from build123d import *

# Parameters (mm, degrees)
SKETCH1_W           = 70.104
SKETCH1_H           = 14.986
BOSS_EXTRUDE1_DEPTH = 21.9964
CUT_EXTRUDE1_DEPTH  = 75.986616306
SKETCH4_R           = 1.5
CUT_EXTRUDE2_DEPTH  = 75.986616306
SKETCH5_R           = 1.27
BOSS_EXTRUDE2_DEPTH = 17.272
BOSS_EXTRUDE3_DEPTH = 14.986
SKETCH7_W           = 11.9888
SKETCH7_H           = 21.9964
BOSS_EXTRUDE4_DEPTH = 0.508
BOSS_EXTRUDE4_TAPER = 45


with BuildPart() as part:
    # Sketch1 → Boss-Extrude1 (new body)
    with BuildSketch(Plane(origin=(0, 0, 0), x_dir=(1, 0, 0), z_dir=(0, 1, 0))):
        with Locations((-35.052, 7.493)):
            Rectangle(SKETCH1_W, SKETCH1_H)
    extrude(amount=BOSS_EXTRUDE1_DEPTH)

    # Sketch3 → Cut-Extrude1 (cut, through all)
    with BuildSketch(Plane.XY):
        with BuildLine():
            Line((-29.337, 13.735160497), (-40.767, 13.735160497))
            ThreePointArc((-40.767, 13.735160497), (-58.1152, 10.9982), (-40.767, 8.261239503))
            Line((-40.767, 8.261239503), (-29.337, 8.261239503))
            ThreePointArc((-29.337, 8.261239503), (-11.9888, 10.9982), (-29.337, 13.735160497))
        make_face()
        Polygon((-58.1152, 21.9964), (-55.5752, 21.3614), (-14.5288, 21.3614), (-11.9888, 21.9964), align=None)
        Polygon((-58.1152, 0), (-55.5752, 0.635), (-14.5288, 0.635), (-11.9888, 0), align=None)
    extrude(amount=-CUT_EXTRUDE1_DEPTH, mode=Mode.SUBTRACT)

    # Sketch4 → Cut-Extrude2 (cut, through all)
    with BuildSketch(Plane(origin=(0, 21.9964, 0), x_dir=(1, 0, 0), z_dir=(0, 1, 0))):
        with Locations(Location((-64.0588, 10.9982, 0), (0, 0, 270))):
            Circle(SKETCH4_R)
        with Locations(Location((-64.0588, 3.9878, 0), (0, 0, 270))):
            Circle(SKETCH4_R)
        with Locations(Location((-6.0452, 3.9878, 0), (0, 0, 90))):
            Circle(SKETCH4_R)
        with Locations(Location((-6.0452, 10.9982, 0), (0, 0, 90))):
            Circle(SKETCH4_R)
    extrude(amount=-CUT_EXTRUDE2_DEPTH, mode=Mode.SUBTRACT)

    # Sketch5 → Boss-Extrude2 (add)
    with BuildSketch(Plane(origin=(0, 0, 0), x_dir=(0, 0, -1), z_dir=(1, 0, 0))):
        with Locations(Location((7.493, 3.23214606, 0), (0, 0, 180))):
            Circle(SKETCH5_R)
    extrude(amount=BOSS_EXTRUDE2_DEPTH)

    # Sketch6 → Boss-Extrude3 (add, through all)
    with BuildSketch(Plane.XY):
        Polygon((-58.1152, 21.9964), (-55.5752, 21.3614), (-14.5288, 21.3614), (-11.9888, 21.9964), (-14.5288, 22.6314), (-55.5752, 22.6314), align=None)
        Polygon((-55.5752, -0.635), (-14.5288, -0.635), (-11.9888, 0), (-14.5288, 0.635), (-55.5752, 0.635), (-58.1152, 0), align=None)
    extrude(amount=-BOSS_EXTRUDE3_DEPTH)

    # Sketch7 → Boss-Extrude4 (add)
    with BuildSketch(Plane(origin=(0, 0, -14.986), x_dir=(-1, 0, 0), z_dir=(0, 0, -1))):
        with Locations((5.9944, 10.9982)):
            Rectangle(SKETCH7_W, SKETCH7_H)
    extrude(amount=BOSS_EXTRUDE4_DEPTH, taper=BOSS_EXTRUDE4_TAPER)


solid = part.part
Geometry: final body of the model. Coordinates: model frame, mm. A direction names the side the tool comes from. Coordinates: 2 decimals unless noted, no trailing zeros. Order: outer loops, then holes, each group sorted by start corner. A loop starts at its lowest first (then second) coordinate and runs counter-clockwise, first axis right, second up.
1) Section A-A (z = -11). Return loops of the section in (x, y) (3 decimals), then the cut area to 3 significant figures.
Result sheet:
outline: (-70.104, 0) - (-65.559, 0) - (-65.559, 21.996) - (-70.104, 21.996) - close; (-62.559, 0) - (-58.115, 0) - (-55.575, -0.635) - (-14.529, -0.635) - (-11.989, 0) - (-7.545, 0) - (-7.545, 21.996) - (-11.989, 21.996) - (-14.529, 22.631) - (-55.575, 22.631) - (-58.115, 21.996) - (-62.559, 21.996) - close; (-4.545, 0) - (0, 0) - (0, 21.996) - (-4.545, 21.996) - close; hole (-40.767, 8.261) - (-29.337, 8.261) arc R8.89 ccw (long way) to (-29.337, 13.735) - (-40.767, 13.735) arc R8.89 ccw (long way) to start
area: 909 mm2
2) Ray query, probe 1 along Z at (x, y) = (-6, 17); probe 2 along X at (y, z) = (20.75, -3.25); probe 3 along Z at (x, y) = (-64.5, 11.5). Return the intervals inside material, ascending.
Result sheet:
probe 1: z = -15.49 to -12.5, -9.5 to -5.49, -2.49 to 0
probe 2: x = -70.1 to -65.36, -62.75 to -7.35, -4.74 to 0
probe 3: z = -14.99 to -12.43, -9.56 to -5.42, -2.55 to 0
3) Set-up query: faces 1 (the flat face through (-6, 21.996, -8)), 2 (the flat face through (-6, 0, -8)), 3 (the flat face through (-64, 0, -8)), 4 (the flat face through (-41, 16, -14.986)), 5 (the flat face through (-35, 8.261, -7)). Return all of +Z, -Z, +X, -X, +Y, -Y with unobstructed straight access to the full face (end or side cutting, diameter ignored); none if empty.
Result sheet:
face 1: +Z, -Z, +X, +Y
face 2: +Z, -Z, +X, -Y
face 3: +Z, -Z, -X, -Y
face 4: -Z, -X, +Y, -Y
face 5: +Z, -Z
4) Section B-B (x = -34). Return loops of the section in (y, z) (3 decimals).
Result sheet:
outline: (-0.635, -14.986) - (8.261, -14.986) - (8.261, 0) - (-0.635, 0) - close; (13.735, -14.986) - (22.631, -14.986) - (22.631, 0) - (13.735, 0) - close
5) Section D-D (z = -7.5). Return loops of the section in (x, y) (3 decimals).
Result sheet:
outline: (-70.104, 0) - (-58.115, 0) - (-55.575, -0.635) - (-14.529, -0.635) - (-11.989, 0) - (0, 0) - (0, 1.962) - (17.272, 1.962) - (17.272, 4.502) - (0, 4.502) - (0, 21.996) - (-11.989, 21.996) - (-14.529, 22.631) - (-55.575, 22.631) - (-58.115, 21.996) - (-70.104, 21.996) - close; hole (-40.767, 8.261) - (-29.337, 8.261) arc R8.89 ccw (long way) to (-29.337, 13.735) - (-40.767, 13.735) arc R8.89 ccw (long way) to start
6) Draft query along Y for faces 6 (the flat face through (-35, 13.735, -7)), 7 (the cylindrical face through (-6.1, 11.2, -9.5)), 8 (the cylindrical face through (8.515, 2.374, -8.429)). Return one class per face: released by +Y, released by -Y, zero draft, split by the parting line, or undercut.
Result sheet:
face 6: undercut
face 7: zero draft
face 8: split by the parting line
7) Section C-C (y = 17.75). Give the number of separate pieces and of enclosed holes in the cut face, then the cut area to 3 significant figures.
Result sheet:
separate pieces: 3
enclosed holes: 4
area: 681 mm2
8) First-contact query: P1, Ø1, axis at x = -30.5, y = 13, coming from the +Z side; P2, Ø5, axis at x = -30.5, y = 9, coming from the -Z side; P3, Ø6, axis at x = -6, z = -5, coming from the +Y side; P4, Ø1.5, axis at y = 10, z = -2.5, coming from the +X side. Flat tips, straight axial feed; report the tip coordinate or a pass-through.
Result sheet:
P1: passes through
P2: stops at z = -14.99
P3: stops at y = 22
P4: stops at x = 0
